from build123d import *

# Parameters (mm, degrees)
SKETCH_1_W             = 103
SKETCH_1_H             = 22
SM_BASE_FLANGE_1_DEPTH = 1.5
OTHER_START            = -11
OTHER_1_DEPTH          = 22
OTHER_1_2_DEPTH        = 22
SKETCH_7_R             = 0.95
SKETCH_7_R_2           = 4
CUT_EXTRUDE_1_DEPTH    = 54.170270292
SKETCH_8_R             = 4
SKETCH_8_R_2           = 0.95
CUT_EXTRUDE_2_DEPTH    = 10


# Read off the part's stored shape, not the designer's step: 绘制的折弯1
# Sheet-metal steps are written as plain solids
with BuildPart() as part:
    # Sketch 1 → 基体-法兰1 (new body)
    with BuildSketch(Plane.XY):
        Rectangle(SKETCH_1_W, SKETCH_1_H)
    extrude(amount=-SM_BASE_FLANGE_1_DEPTH)

    # Other 1 outline → Other 1 (cut)
    with BuildSketch(Plane(origin=(0, 0, 0), x_dir=(1, 0, 0), z_dir=(0, 1, 0)).offset(OTHER_START)):
        with BuildLine():
            ThreePointArc((-20.611823856, 0), (-19.795164082, 1.086838938), (-18.5, 1.5))
            Line((-18.5, 1.5), (-51.5, 1.5))
            Line((-51.5, 1.5), (-51.5, 0))
            Line((-51.5, 0), (-20.611823856, 0))
        make_face()
        with BuildLine():
            Line((51.5, 1.5), (18.5, 1.5))
            ThreePointArc((18.5, 1.5), (19.795164082, 1.086838938), (20.611823856, 0))
            Line((20.611823856, 0), (51.5, 0))
            Line((51.5, 0), (51.5, 1.5))
        make_face()
    extrude(amount=OTHER_1_DEPTH, mode=Mode.SUBTRACT)

    # Other 1 2 outline → Other 1 2 (add)
    with BuildSketch(Plane(origin=(0, 0, 0), x_dir=(1, 0, 0), z_dir=(0, 1, 0)).offset(OTHER_START)):
        with BuildLine():
            Line((-18.5, 0), (-20.611823856, 0))
            ThreePointArc((-20.611823856, 0), (-20.705185343, -0.363053267), (-20.7366, -0.7366))
            Line((-20.7366, -0.7366), (-20.7366, -31.401454181))
            Line((-20.7366, -31.401454181), (-19.2366, -31.401454181))
            Line((-19.2366, -31.401454181), (-19.2366, -0.7366))
            ThreePointArc((-19.2366, -0.7366), (-19.020854855, -0.215745145), (-18.5, 0))
        make_face()
        with BuildLine():
            ThreePointArc((20.7366, -0.7366), (20.705185343, -0.363053267), (20.611823856, 0))
            Line((20.611823856, 0), (18.5, 0))
            ThreePointArc((18.5, 0), (19.020854855, -0.215745145), (19.2366, -0.7366))
            Line((19.2366, -0.7366), (19.2366, -31.401454181))
            Line((19.2366, -31.401454181), (20.7366, -31.401454181))
            Line((20.7366, -31.401454181), (20.7366, -0.7366))
        make_face()
    extrude(amount=OTHER_1_2_DEPTH)

    # 草图7 → 切除-拉伸1 (cut, through all)
    with BuildSketch(Plane.ZY.offset(20.7366)):
        with Locations((20.401454181, 8)):
            Circle(SKETCH_7_R)
        with Locations((12.401454181, 0)):
            Circle(SKETCH_7_R)
        with Locations((20.401454181, 0)):
            Circle(SKETCH_7_R_2)
        with Locations((28.401454181, 0)):
            Circle(SKETCH_7_R)
        with Locations((20.401454181, -8)):
            Circle(SKETCH_7_R)
        with BuildLine():
            ThreePointArc((20.401454181, 11), (28.179628774, 7.778174593), (31.401454181, 0))
            Line((31.401454181, 0), (31.401454181, 11))
            Line((31.401454181, 11), (20.401454181, 11))
        make_face()
        with BuildLine():
            Line((31.401454181, -11), (31.401454181, 0))
            ThreePointArc((31.401454181, 0), (28.179628774, -7.778174593), (20.401454181, -11))
            Line((20.401454181, -11), (31.401454181, -11))
        make_face()
    extrude(amount=-CUT_EXTRUDE_1_DEPTH, mode=Mode.SUBTRACT)

    # 草图8 → 切除-拉伸2 (cut)
    with BuildSketch(Plane.XY):
        Circle(SKETCH_8_R)
        with Locations((0, 8)):
            Circle(SKETCH_8_R_2)
        with Locations((8, 0)):
            Circle(SKETCH_8_R_2)
        with Locations((0, -8)):
            Circle(SKETCH_8_R_2)
        with Locations((-8, 0)):
            Circle(SKETCH_8_R_2)
    extrude(amount=-CUT_EXTRUDE_2_DEPTH, mode=Mode.SUBTRACT)


solid = part.part
Read the model definition and answer for the solid it produces. Units are mm, in the model's axes. A direction names the side the tool comes from. Coordinates: 2 decimals unless noted, no trailing zeros. Loops run counter-clockwise (first coordinate to the right, second up) from the corner with the lowest first, then second, coordinate; pieces in that order, holes last. Notation, with made-up numbers: (37, -15) -> (83, -15) arc R28 cw to (83, 3) -> close; hole circle Ø3 at (84, 73.5). An arc over 180 degrees is marked (long way). Write item = value, one per line. Start each with the question number.
1) The mould has two halves that part along X. Classify faces 3 (the face through (-20.737, 0, 16)), 4 (the face through (-0.124, 8.942, -0.74)), 5 (the face through (20.737, 0, 16)), 6 (the face through (-20, 8.64, 19.7)): pulls with the +X half, pulls with the -X half, needs draft (parallel to the pull), parting line crosses it, or undercut.
2) The part is cut by section B-B, the plane z = 9. Determine the outline of the cut face in (x, y), plus the area to 3 significant figures.
3) For faces 1 (the face through (-19.237, 0, 16)), 2 (the face through (19.976, -3.549, 22.247)), determine the directions among +Z, -Z, +X, -X, +Y, -Y from which every point of the face is accessible in a straight line to the end or side of a thin tool.
4) The part is cut by section C-C, the plane x = -8. Determine the outline of the cut face in (y, z), plus the area to 4 significant figures.
5) Given P1, Ø11, axis at x = 0.5, y = 3, coming from the +Z side; P2, Ø8, axis at x = -15, y = 2, coming from the +Z side, each flat-ended and moving along its own axis, determine where each tip first touches the part or whether it passes through.
6) Find the intervals of material crossed by L1, parallel to Y at x = 0, z = -1; L2, parallel to X at y = -5, z = 21.5; L3, parallel to Z at x = 13.5, y = 4.5, in increasing order. Write a range as from..to.
7) The part is cut by section D-D, the plane y = 1.5. Determine the outline of the cut face in (x, z), plus the area to 3 significant figures.
8) The part is cut by section A-A, the plane x = 0. Determine the outline of the cut face in (y, z), plus the area to 3 significant figures.
Result:
q1.face_3 = pulls with the -X half
q1.face_4 = undercut
q1.face_5 = pulls with the +X half
q1.face_6 = needs draft
q2.outline = (-20.74, -11) -> (-19.24, -11) -> (-19.24, 11) -> (-20.74, 11) -> close; (19.24, -11) -> (20.74, -11) -> (20.74, 11) -> (19.24, 11) -> close
q2.area = 66.0 mm²
q3.face_1 = +Z, +Y, -Y
q3.face_2 = +X, -X
q4.outline = (-11, -1.5) -> (-0.95, -1.5) -> (-0.95, 0) -> (-11, 0) -> close; (0.95, -1.5) -> (11, -1.5) -> (11, 0) -> (0.95, 0) -> close
q4.area = 30.15 mm²
q5.P1 = 0
q5.P2 = 0.2
q6.L1 = -11..-8.95, -7.05..-4, 4..7.05, 8.95..11
q6.L2 = -20.74..-19.24, 19.24..20.74
q6.L3 = -1.5..0
q7.outline = (-20.74, 0.74) arc R2.24 ccw to (-18.5, -1.5) -> (-3.71, -1.5) -> (-3.71, 0) -> (-18.5, 0) arc R0.74 cw to (-19.24, 0.74) -> (-19.24, 16.69) -> (-20.74, 16.69) -> close; (-20.74, 24.11) -> (-19.24, 24.11) -> (-19.24, 31.3) -> (-20.74, 31.3) -> close; (3.71, -1.5) -> (18.5, -1.5) arc R2.24 ccw to (20.74, 0.74) -> (20.74, 16.69) -> (19.24, 16.69) -> (19.24, 0.74) arc R0.74 cw to (18.5, 0) -> (3.71, 0) -> close; (19.24, 24.11) -> (20.74, 24.11) -> (20.74, 31.3) -> (19.24, 31.3) -> close
q7.area = 121 mm²
q8.outline = (-11, -1.5) -> (-8.95, -1.5) -> (-8.95, 0) -> (-11, 0) -> close; (-7.05, -1.5) -> (-4, -1.5) -> (-4, 0) -> (-7.05, 0) -> close; (4, -1.5) -> (7.05, -1.5) -> (7.05, 0) -> (4, 0) -> close; (8.95, -1.5) -> (11, -1.5) -> (11, 0) -> (8.95, 0) -> close
q8.area = 15.3 mm²
